Answer from the drawing. Dimensions are ordinates in mm from the lowest x, y and z of the part. Give positions to 0.01 mm unless a question says otherwise; leave off trailing zeros. Write each loop counter-clockwise with the first axis right and the second up, starting at its lowest first coordinate (ties: lowest second). Pieces come first, ordered by that corner, then holes. Notation, with made-up numbers: M -15.5,56.5 L 32.5,56.5 A21 cw 32.5,85.5 Z; hole C 78,-1.75 d1. An arc over 180 degrees is marked long. Put each result on its own line as item: value.
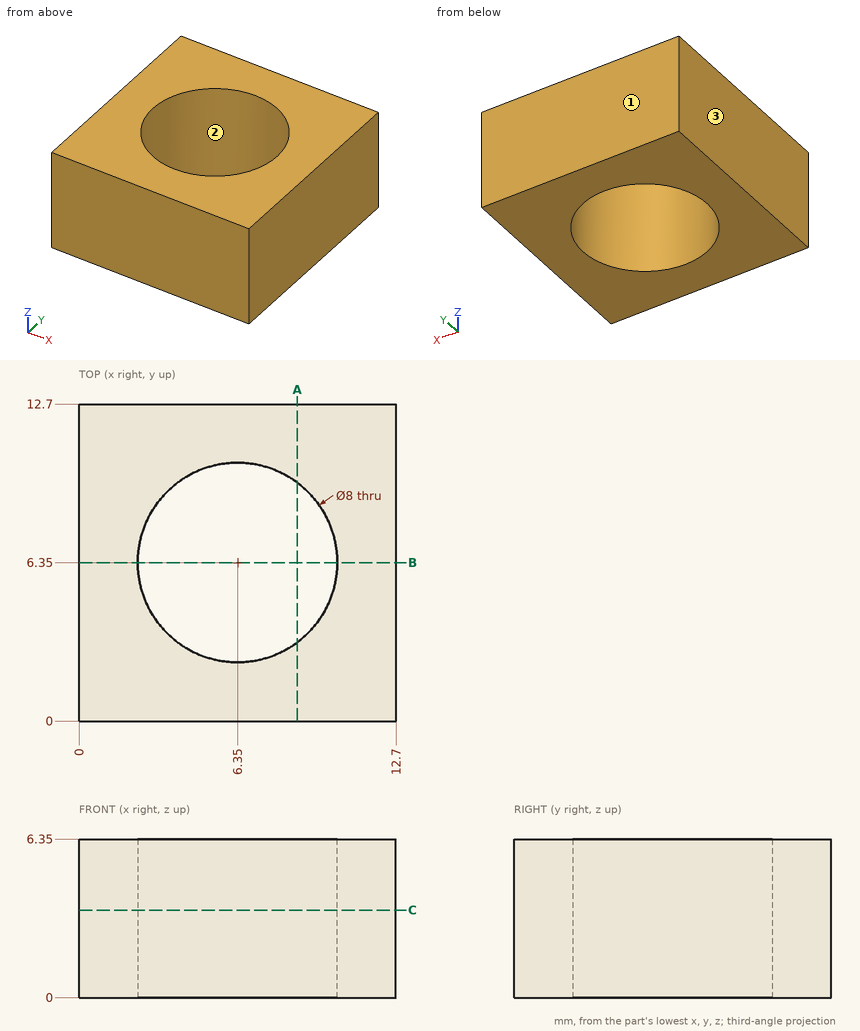
(1) For a pull along X with two mould halves and no side action, classify the marked faces 1, 2 and 3 as +X half, -X half, draft (parallel to the pull), parting line (faces both ways), or undercut.
Result:
face 1: draft
face 2: undercut
face 3: -X half
(2) Section B-B on y = 6.35 is taken. Determine the outline of the cut face in (x, z).
Result:
outline: M 0,0 L 2.35,0 L 2.35,6.35 L 0,6.35 Z; M 10.35,0 L 12.7,0 L 12.7,6.35 L 10.35,6.35 Z
(3) Straight lines are drawn through the part: line 1 along X through (y, z) = (6.35, 4.75); line 2 along X through (y, z) = (2.75, 4.75). For each, find the intervals that lie inside material, in ascending order. Write a range as from..to.
Result:
line 1: x = 0..2.35, 10.35..12.7
line 2: x = 0..4.61, 8.09..12.7
(4) Section C-C on z = 3.5 is taken. Determine the outline of the cut face in (x, y).
Result:
outline: M 0,0 L 12.7,0 L 12.7,12.7 L 0,12.7 Z; hole C 6.35,6.35 d8
(5) Given pin 1 Ø6.5 at (x, y) = (6.35, 6.35) entering from +Z, flat-ended and moving along its own axis, determine where the tip first touches the part or whether it passes through.
Result:
pin 1: passes through
(6) Section A-A on x = 8.75 is taken. Determine the outline of the cut face in (y, z).
Result:
outline: M 0,0 L 3.15,0 L 3.15,6.35 L 0,6.35 Z; M 9.55,0 L 12.7,0 L 12.7,6.35 L 9.55,6.35 Z
